from build123d import *

# Parameters (mm, degrees)
F1_DEPTH = 25.4
F3_DEPTH = 3.048
F4_R     = 15.0876
F5_DEPTH = 28.449


with BuildPart() as f1:
    # F0 (on Front) → F1 (new body)
    with BuildSketch(Plane.XZ):
        Polygon((11.152286, 26.924), (-11.152286, 26.924), (-26.924, 11.152286), (-26.924, -11.152286), (-11.152286, -26.924), (11.152286, -26.924), (26.924, -11.152286), (26.924, 11.152286), align=None)
    extrude(amount=F1_DEPTH)

    # F2 (on face) → F3 (join)
    with BuildSketch(Plane.XZ.offset(25.4)):
        Polygon((11.80985, 28.5115), (-11.80985, 28.5115), (-28.5115, 11.80985), (-28.5115, -11.80985), (-11.80985, -28.5115), (11.80985, -28.5115), (28.5115, -11.80985), (28.5115, 11.80985), align=None)
    extrude(amount=F3_DEPTH)

    # F4 (on face) → F5 (cut, through all)
    with BuildSketch(Plane.XZ.offset(28.448)):
        Circle(F4_R)
    extrude(amount=-F5_DEPTH, mode=Mode.SUBTRACT)


solid = f1.part
Geometry check sheet. Reference: the model listing, model coordinates, mm. A direction names the side the tool comes from. Coordinates: 2 decimals unless noted, no trailing zeros. Order: outer loops, then holes, each group sorted by start corner. A loop starts at its lowest first (then second) coordinate and runs counter-clockwise, first axis right, second up. Notation, with made-up numbers: (46.25, 55) -> (84.25, 55) arc R15 ccw to (84.25, 79) -> close; hole circle Ø6 at (65, 38). An arc over 180 degrees is marked (long way). Use a Markdown table: item, result. Add a question column.
1. Cross-section at C-C (y = -26.25). Enter the section's corners in (x, z), and give its area (3 significant figures).
2. Go/stop test with flat-tipped pins: pin 1 Ø6.5 at (x, y) = (2, -16.5) entering from +Z; pin 2 Ø6.5 at (x, y) = (5, -10) entering from -Z; pin 3 Ø6 at (x, y) = (14.5, -20.5) entering from -Z. Record where each tip stops, or that it passes through.
3. Mould release check, pull along Z, two halves, no side actions. Record for faces 6 (the face through (-11.973, -14.423, -9.181)), 7 (the face through (20.28, -26.9, 20.04)), 8 (the face through (-13, -28.448, 13)): pulls with the +Z half, pulls with the -Z half, needs draft (parallel to the pull), parting line crosses it, or undercut.
4. Cross-section at B-B (x = 0). Enter the section's corners in (y, z), and give its area (3 significant figures).
5. Cross-section at D-D (y = -14.25). Enter the section's corners in (x, z), and give its area (3 significant figures).
6. Material ranges on L1, parallel to Z at x = 0, y = -5.75; L2, parallel to X at y = -12, z = 0.5; L3, parallel to Z at x = -9, y = -16.75, recorded low to high.
7. Cross-section at A-A (z = 0). Enter the section's corners in (x, y), and give its area (3 significant figures).
8. Set-up check for faces 1 (the face through (26.924, -13, 0)), 2 (the face through (19.149, -12.522, 18.928)), 3 (the face through (0, -13, 26.924)), 4 (the face through (-26.924, -13, 0)), 5 (the face through (-0.1, -25.4, -27.3)): record each of +Z, -Z, +X, -X, +Y, -Y from which the full face is reachable in a straight line by a thin tool's end or side.
Filled sheet:
| question | item | result |
|---|---|---|
| 1 | outline | (-28.51, -11.81) -> (-11.81, -28.51) -> (11.81, -28.51) -> (28.51, -11.81) -> (28.51, 11.81) -> (11.81, 28.51) -> (-11.81, 28.51) -> (-28.51, 11.81) -> close; hole circle Ø30.18 at (0, 0) |
| 1 | area | 1,980 mm2 |
| 2 | pin 1 | z = 26.92 |
| 2 | pin 2 | z = -26.92 |
| 2 | pin 3 | z = -26.58 |
| 3 | face 6 | undercut |
| 3 | face 7 | pulls with the +Z half |
| 3 | face 8 | needs draft |
| 4 | outline | (-28.45, -28.51) -> (-25.4, -28.51) -> (-25.4, -26.92) -> (0, -26.92) -> (0, -15.09) -> (-28.45, -15.09) -> close; (-28.45, 15.09) -> (0, 15.09) -> (0, 26.92) -> (-25.4, 26.92) -> (-25.4, 28.51) -> (-28.45, 28.51) -> close |
| 4 | area | 683 mm2 |
| 5 | outline | (-26.92, -11.15) -> (-11.15, -26.92) -> (11.15, -26.92) -> (26.92, -11.15) -> (26.92, 11.15) -> (11.15, 26.92) -> (-11.15, 26.92) -> (-26.92, 11.15) -> close; hole circle Ø30.18 at (0, 0) |
| 5 | area | 1,690 mm2 |
| 6 | L1 | -26.92 to -15.09, 15.09 to 26.92 |
| 6 | L2 | -26.92 to -15.08, 15.08 to 26.92 |
| 6 | L3 | -26.92 to -12.11, 12.11 to 26.92 |
| 7 | outline | (-28.51, -28.45) -> (-15.09, -28.45) -> (-15.09, 0) -> (-26.92, 0) -> (-26.92, -25.4) -> (-28.51, -25.4) -> close; (15.09, -28.45) -> (28.51, -28.45) -> (28.51, -25.4) -> (26.92, -25.4) -> (26.92, 0) -> (15.09, 0) -> close |
| 7 | area | 683 mm2 |
| 8 | face 1 | +Z, -Z, +X, +Y |
| 8 | face 2 | +Z, +X, +Y |
| 8 | face 3 | +Z, +X, -X, +Y |
| 8 | face 4 | +Z, -Z, -X, +Y |
| 8 | face 5 | +Y |
